from build123d import *

# Parameters (mm, degrees)
SKETCH1_W  = 42.2
SKETCH1_H  = 36.76
SKETCH1_R  = 3.15
BASE_DEPTH = 2
SKETCH3_W  = 36.76
SKETCH3_H  = 33.9
SKETCH3_R  = 3.225
TAB_DEPTH  = 2


with BuildPart() as part:
    # Sketch1 → Base (new body)
    with BuildSketch(Plane(origin=(0, 0, 0), x_dir=(1, 0, 0), z_dir=(0, 1, 0))):
        Rectangle(SKETCH1_W, SKETCH1_H)
        with Locations((14.99, 12.1)):
            Circle(SKETCH1_R, mode=Mode.SUBTRACT)
        with Locations((14.99, -9.9)):
            Circle(SKETCH1_R, mode=Mode.SUBTRACT)
    extrude(amount=BASE_DEPTH)

    # Sketch3 → Tab (add)
    with BuildSketch(Plane.ZY.offset(21.1)):
        with Locations((0, 16.95)):
            Rectangle(SKETCH3_W, SKETCH3_H)
        with Locations((-3.225, 26.835)):
            Circle(SKETCH3_R, mode=Mode.SUBTRACT)
        with Locations((9.295, 26.835)):
            Circle(SKETCH3_R, mode=Mode.SUBTRACT)
    extrude(amount=-TAB_DEPTH)


solid = part.part
For this review, take the finished solid that the model builds, in its own axes (mm). A direction names the side the tool comes from. Coordinates: 2 decimals unless noted, no trailing zeros. Loops run counter-clockwise (first coordinate to the right, second up) from the corner with the lowest first, then second, coordinate; pieces in that order, holes last. Notation, with made-up numbers: (79.25, -4) - (116.25, -4) arc R20 ccw to (116.25, 28) - close; hole circle Ø5 at (82, 5). An arc over 180 degrees is marked (long way). Use a Markdown table: item, result. Add a question column.
Item 1: For line 1 (X direction, y = 0.75, z = 9.9); line 2 (X direction, y = 32, z = -2); line 3 (Y direction, x = 2, z = 1), list the stretches that pass through material, from the lowest coordinate up.
Item 2: Mouldability with a two-part tool opening along Z and no side actions: class faces 3 (the face through (0, 0, 0)), 4 (the face through (12.49, 0.986, 11.817)), 5 (the face through (-20.114, 30.033, -3.645)), 6 (the face through (-6.4, 1.8, 18.38)) as pulls with the +Z half, pulls with the -Z half, needs draft (parallel to the pull), parting line crosses it, or undercut.
Item 3: Tool access review of faces 1 (the face through (-21.1, 17, 0)), 2 (the face through (-19.1, 18, 0)): name each direction out of +Z, -Z, +X, -X, +Y, -Y from which nothing blocks a thin tool from reaching the whole face with its end or side.
Item 4: We need section B-B (x = 14.99). Give the boundary of the cut face in (y, z), and give its area (3 significant figures).
Item 5: We need section D-D (z = 4.5). Give the boundary of the cut face in (x, y), and give its area (3 significant figures).
Item 6: We need section C-C (y = 25.5). Give the boundary of the cut face in (x, z), and give its area (3 significant figures).
Item 7: Insertion check: pin 1 Ø5 at (x, z) = (14.99, 9.9) entering from -Y; pin 2 Ø10 at (x, z) = (15, -9) entering from +Y; pin 3 Ø8.5 at (y, z) = (26.835, 9.295) entering from +X. Each pin has a flat end and moves straight along its axis. Give the tip position at first contact, or say it passes through.
Item 8: We need section A-A (z = -12.1). Give the boundary of the cut face in (x, y), and give its area (3 significant figures).
Results list:
| question | item | result |
|---|---|---|
| 1 | line 1 | x = -21.1 to 11.84, 18.14 to 21.1 |
| 1 | line 2 | x = -21.1 to -19.1 |
| 1 | line 3 | y = 0 to 2 |
| 2 | face 3 | needs draft |
| 2 | face 4 | undercut |
| 2 | face 5 | undercut |
| 2 | face 6 | pulls with the +Z half |
| 3 | face 1 | +Z, -Z, -X, +Y, -Y |
| 3 | face 2 | +Z, -Z, +X, +Y |
| 4 | outline | (0, -18.38) - (2, -18.38) - (2, -15.25) - (0, -15.25) - close; (0, -8.95) - (2, -8.95) - (2, 6.75) - (0, 6.75) - close; (0, 13.05) - (2, 13.05) - (2, 18.38) - (0, 18.38) - close |
| 4 | area | 48.3 mm^2 |
| 5 | outline | (-21.1, 0) - (21.1, 0) - (21.1, 2) - (-19.1, 2) - (-19.1, 33.9) - (-21.1, 33.9) - close |
| 5 | area | 148 mm^2 |
| 6 | outline | (-21.1, -18.38) - (-19.1, -18.38) - (-19.1, -6.16) - (-21.1, -6.16) - close; (-21.1, -0.29) - (-19.1, -0.29) - (-19.1, 6.36) - (-21.1, 6.36) - close; (-21.1, 12.23) - (-19.1, 12.23) - (-19.1, 18.38) - (-21.1, 18.38) - close |
| 6 | area | 50.0 mm^2 |
| 7 | pin 1 | passes through |
| 7 | pin 2 | stops at y = 2 |
| 7 | pin 3 | stops at x = -19.1 |
| 8 | outline | (-21.1, 0) - (11.84, 0) - (11.84, 2) - (-19.1, 2) - (-19.1, 33.9) - (-21.1, 33.9) - close; (18.14, 0) - (21.1, 0) - (21.1, 2) - (18.14, 2) - close |
| 8 | area | 136 mm^2 |
